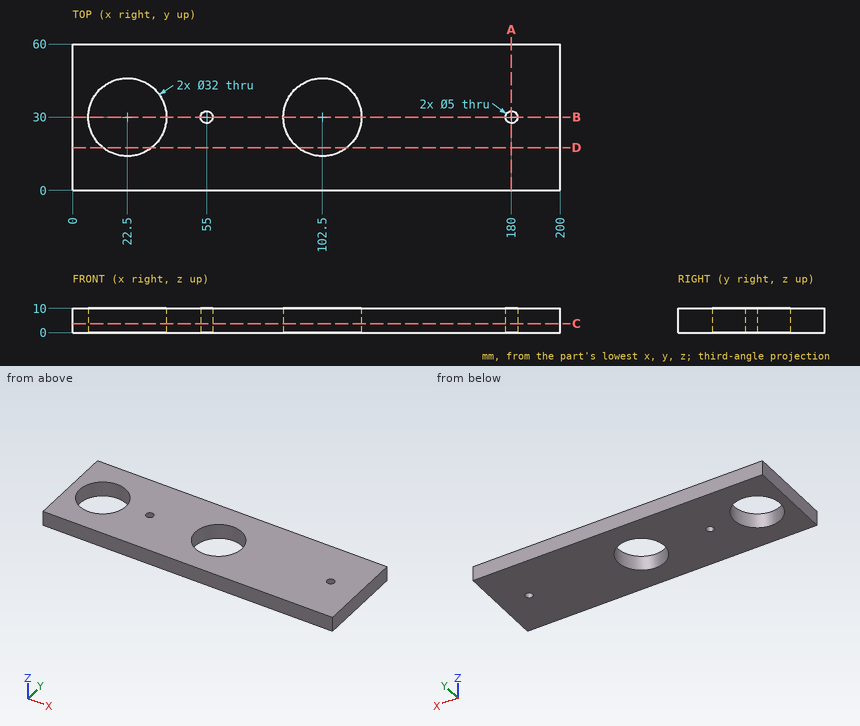
The figure shows three views and two pictorial views of one solid part (mm, origin at its lowest corner). Answer the questions. Give positions to 0.01 mm unless a question says otherwise; leave off trailing zeros. Order: outer loops, then holes, each group sorted by start corner. A loop starts at its lowest first (then second) coordinate and runs counter-clockwise, first axis right, second up. Notation, with made-up numbers: (17.5, 20) -> (42.5, 20) arc R37 cw to (42.5, 56) -> close; hole circle Ø11 at (-31, -34). An arc over 180 degrees is marked (long way). Write each question's results on one line, items separated by ' | '.
Q1. The part is cut by section B-B, the plane y = 30. Give the vertices of the cut face in (x, z), and give its area (3 significant figures).
Checked values:
outline: (0, 0) -> (6.5, 0) -> (6.5, 10) -> (0, 10) -> close; (38.5, 0) -> (52.5, 0) -> (52.5, 10) -> (38.5, 10) -> close; (57.5, 0) -> (86.5, 0) -> (86.5, 10) -> (57.5, 10) -> close; (118.5, 0) -> (177.5, 0) -> (177.5, 10) -> (118.5, 10) -> close; (182.5, 0) -> (200, 0) -> (200, 10) -> (182.5, 10) -> close | area: 1,260 mm^2
Q2. The part is cut by section A-A, the plane x = 180. Give the vertices of the cut face in (y, z), and give its area (3 significant figures).
Checked values:
outline: (0, 0) -> (27.5, 0) -> (27.5, 10) -> (0, 10) -> close; (32.5, 0) -> (60, 0) -> (60, 10) -> (32.5, 10) -> close | area: 550 mm^2
Q3. This flat-tipped pin is pushed along its axis until it touches: P1, Ø4.5, axis at x = 55, y = 30, coming from the -Z side. Where does it stop, or does it pass through?
Checked values:
P1: passes through
Q4. Straight lines are drawn through the part: probe 1 along Y at (x, z) = (102.5, 5.25); probe 2 along X at (y, z) = (25.5, 2); probe 3 along X at (y, z) = (24.5, 3.75). For each, find the intervals that lie inside material, in ascending order. Write a range as from..to.
Checked values:
probe 1: y = 0..14, 46..60 | probe 2: x = 0..7.15, 37.85..87.15, 117.85..200 | probe 3: x = 0..7.48, 37.52..87.48, 117.52..200
Q5. The part is cut by section C-C, the plane z = 3.75. Give the vertices of the cut face in (x, y).
Checked values:
outline: (0, 0) -> (200, 0) -> (200, 60) -> (0, 60) -> close; hole circle Ø32 at (22.5, 30); hole circle Ø5 at (55, 30); hole circle Ø32 at (102.5, 30); hole circle Ø5 at (180, 30)
Q6. The part is cut by section D-D, the plane y = 17.5. Give the vertices of the cut face in (x, z), and give its area (3 significant figures).
Checked values:
outline: (0, 0) -> (12.51, 0) -> (12.51, 10) -> (0, 10) -> close; (32.49, 0) -> (92.51, 0) -> (92.51, 10) -> (32.49, 10) -> close; (112.49, 0) -> (200, 0) -> (200, 10) -> (112.49, 10) -> close | area: 1,600 mm^2
